from build123d import *
from OCP.BRepFilletAPI import BRepFilletAPI_MakeChamfer

# Parameters (mm, degrees)
SKETCH1_W           = 6.858
SKETCH1_H           = 5.334
BOSS_EXTRUDE1_DEPTH = 4.826
SKETCH2_W           = 1.524
SKETCH2_H           = 1.524
BOSS_EXTRUDE2_DEPTH = 4.826
CHAMFER1_SIZE       = 0.9398
CHAMFER1_SIZE2      = 0.542593783
BOSS_EXTRUDE3_START = -3.048
SKETCH3_W           = 0.720393783
SKETCH3_H           = 1.524
SKETCH3_W_2         = 0.981406217
SKETCH3_W_3         = 1.524
SKETCH3_H_2         = 1.1176
SKETCH3_H_3         = 0.5842
SKETCH3_H_4         = 0.981406217
SKETCH3_H_5         = 0.720393783
BOSS_EXTRUDE3_DEPTH = 0.2032
FILLET2_R           = 0.0508
FILLET3_R           = 0.635
FILLET6_R           = 1.27
SKETCH4_W           = 3.2766
SKETCH4_H           = 3.2258
CUT_EXTRUDE1_DEPTH  = 2.032


with BuildPart() as part:
    # Sketch1 → Boss-Extrude1 (new body)
    with BuildSketch(Plane(origin=(0, 0, 0), x_dir=(1, 0, 0), z_dir=(0, 1, 0))):
        Rectangle(SKETCH1_W, SKETCH1_H)
    extrude(amount=BOSS_EXTRUDE1_DEPTH)

    # Sketch2 → Boss-Extrude2 (add)
    with BuildSketch(Plane(origin=(0, 4.826, 0), x_dir=(1, 0, 0), z_dir=(0, 1, 0))):
        Rectangle(SKETCH2_W, SKETCH2_H)
        with Locations((1.524, 0)):
            Rectangle(SKETCH2_W, SKETCH2_H)
        with Locations((0, 1.524)):
            Rectangle(SKETCH2_W, SKETCH2_H)
        with Locations((-1.524, 0)):
            Rectangle(SKETCH2_W, SKETCH2_H)
        with Locations((0, -1.524)):
            Rectangle(SKETCH2_W, SKETCH2_H)
    extrude(amount=BOSS_EXTRUDE2_DEPTH)

    # Chamfer1: one chamfer whose edges measure the first distance from different faces: ONE call of the kernel's chamfer builder (chamfer() names one face for all edges)
    chamfer1_edges_1 = [part.edges().sort_by_distance(p)[0] for p in [
        (2.286, 9.652, 0),
    ]]
    chamfer1_side_1 = [part.faces().sort_by_distance(p)[0] for p in [
        (2.286, 7.239, 0),
    ]]
    chamfer1_edges_2 = [part.edges().sort_by_distance(p)[0] for p in [
        (0, 9.652, -2.286),
    ]]
    chamfer1_side_2 = [part.faces().sort_by_distance(p)[0] for p in [
        (0, 9.652, 0),
    ]]
    chamfer1_edges_3 = [part.edges().sort_by_distance(p)[0] for p in [
        (-2.286, 9.652, 0),
    ]]
    chamfer1_side_3 = [part.faces().sort_by_distance(p)[0] for p in [
        (-2.286, 7.239, 0),
    ]]
    chamfer1_edges_4 = [part.edges().sort_by_distance(p)[0] for p in [
        (0, 9.652, 2.286),
    ]]
    chamfer1_side_4 = [part.faces().sort_by_distance(p)[0] for p in [
        (0, 7.239, 2.286),
    ]]
    chamfer1 = BRepFilletAPI_MakeChamfer(part.part.solid().wrapped)
    for e in chamfer1_edges_1:
        chamfer1.Add(CHAMFER1_SIZE, CHAMFER1_SIZE2, e.wrapped, chamfer1_side_1[0].wrapped)  # the first distance lies on this face
    for e in chamfer1_edges_2:
        chamfer1.Add(CHAMFER1_SIZE, CHAMFER1_SIZE2, e.wrapped, chamfer1_side_2[0].wrapped)  # the first distance lies on this face
    for e in chamfer1_edges_3:
        chamfer1.Add(CHAMFER1_SIZE, CHAMFER1_SIZE2, e.wrapped, chamfer1_side_3[0].wrapped)  # the first distance lies on this face
    for e in chamfer1_edges_4:
        chamfer1.Add(CHAMFER1_SIZE, CHAMFER1_SIZE2, e.wrapped, chamfer1_side_4[0].wrapped)  # the first distance lies on this face
    add(Compound.cast(chamfer1.Shape()), mode=Mode.REPLACE)

    # Sketch3 → Boss-Extrude3 (add)
    with BuildSketch(Plane(origin=(0, 9.652, 0), x_dir=(1, 0, 0), z_dir=(0, 1, 0)).offset(BOSS_EXTRUDE3_START)):
        with Locations((2.103603109, 0)):
            Rectangle(SKETCH3_W, SKETCH3_H)
        with Locations((1.252703108, 0)):
            Rectangle(SKETCH3_W_2, SKETCH3_H)
        with Locations((0, 1.905)):
            Rectangle(SKETCH3_W_3, SKETCH3_H_2)
        with Locations((0, 1.0541)):
            Rectangle(SKETCH3_W_3, SKETCH3_H_3)
        Rectangle(SKETCH3_W_3, SKETCH3_H)
        with Locations((-1.252703108, 0)):
            Rectangle(SKETCH3_W_2, SKETCH3_H)
        with Locations((-2.103603109, 0)):
            Rectangle(SKETCH3_W, SKETCH3_H)
        with Locations((0, -1.252703108)):
            Rectangle(SKETCH3_W_3, SKETCH3_H_4)
        with Locations((0, -2.103603109)):
            Rectangle(SKETCH3_W_3, SKETCH3_H_5)
    extrude(amount=BOSS_EXTRUDE3_DEPTH)

    # Fillet2
    fillet2_edges = [part.edges().sort_by_distance(p)[0] for p in [
        (-2.4638, 6.8072, 0),
        (0, 6.8072, 2.4638),
        (2.4638, 6.604, 0),
        (2.4638, 6.8072, 0),
        (2.4638, 6.7056, 0.762),
        (2.4638, 6.7056, -0.762),
        (0, 6.8072, -2.4638),
        (0.762, 6.7056, -2.4638),
        (-0.762, 6.7056, -2.4638),
        (-2.4638, 6.604, 0),
        (-2.4638, 6.7056, -0.762),
        (0, 6.604, 2.4638),
        (-0.762, 6.7056, 2.4638),
        (0, 6.604, -2.4638),
        (-2.4638, 6.7056, 0.762),
        (0.762, 6.7056, 2.4638),
    ]]
    fillet(fillet2_edges, radius=FILLET2_R)

    # Fillet3
    fillet3_edges = [part.edges().sort_by_distance(p)[0] for p in [
        (3.429, 2.413, 2.667),
        (-3.429, 2.413, -2.667),
        (3.429, 2.413, -2.667),
    ]]
    fillet(fillet3_edges, radius=FILLET3_R)

    # Fillet6
    fillet6_edges = [part.edges().sort_by_distance(p)[0] for p in [
        (-3.429, 2.413, 2.667),
    ]]
    fillet(fillet6_edges, radius=FILLET6_R)

    # Sketch4 → Cut-Extrude1 (cut)
    with BuildSketch(Plane.XZ):
        Rectangle(SKETCH4_W, SKETCH4_H)
    extrude(amount=-CUT_EXTRUDE1_DEPTH, mode=Mode.SUBTRACT)


solid = part.part
Verification items for the finished model (mm, model axes). A direction names the side the tool comes from. Coordinates: 2 decimals unless noted, no trailing zeros. Loops run counter-clockwise (first coordinate to the right, second up) from the corner with the lowest first, then second, coordinate; pieces in that order, holes last. Notation, with made-up numbers: M 50,77.5 L 55,77.5 A27 cw 55,98.5 Z; hole C -7,49 d3. An arc over 180 degrees is marked long. One line per item, written item: value.
1. Mould release check, pull along Y, two halves, no side actions. Record for faces 1 (the flat face through (2.286, 6, 0)), 2 (the flat face through (-3.429, 2, 0)), 3 (the flat face through (0, 0, -2)): pulls with the +Y half, pulls with the -Y half, needs draft (parallel to the pull), parting line crosses it, or undercut.
Answers follow:
face 1: undercut
face 2: needs draft
face 3: pulls with the -Y half
2. Section check B-B on x = -0.25. Record the cut outline in (y, z).
Answers follow:
outline: M 0,-2.67 L 4.83,-2.67 L 4.83,-2.29 L 6.6,-2.29 L 6.6,-2.41 A0.05 ccw 6.65,-2.46 L 6.76,-2.46 A0.05 ccw 6.81,-2.41 L 6.81,-2.29 L 9.11,-2.29 L 9.65,-1.35 L 9.65,1.74 L 8.71,2.29 L 6.81,2.29 L 6.81,2.41 A0.05 ccw 6.76,2.46 L 6.65,2.46 A0.05 ccw 6.6,2.41 L 6.6,2.29 L 4.83,2.29 L 4.83,2.67 L 0,2.67 L 0,1.61 L 2.03,1.61 L 2.03,-1.61 L 0,-1.61 Z
3. Gauge pin test, flat ends, axial feed: P1, Ø3, axis at x = 0, z = -0.5, coming from the -Y side; P2, Ø0.5, axis at x = -2, y = 7, coming from the +Z side; P3, Ø1.2, axis at y = 6, z = -2, coming from the +X side; P4, Ø0.5, axis at x = 0, y = 6, coming from the +Z side. Record the tip position at first contact, or that the pin passes through.
Answers follow:
P1: y = 0
P2: z = 0.76
P3: x = 0.76
P4: z = 2.29
4. Section check D-D on y = 6.5. Record the cut outline in (x, z).
Answers follow:
outline: M -2.29,-0.76 L -0.76,-0.76 L -0.76,-2.29 L 0.76,-2.29 L 0.76,-0.76 L 2.29,-0.76 L 2.29,0.76 L 0.76,0.76 L 0.76,2.29 L -0.76,2.29 L -0.76,0.76 L -2.29,0.76 Z
5. Material ranges on line 1 along X through (y, z) = (1.75, -0.7); line 2 along Y through (x, z) = (-1.5, -1.75); line 3 along Z through (x, y) = (1, 5.5), recorded low to high. Write a range as from..to.
Answers follow:
line 1: -3.43..-1.64, 1.64..3.43
line 2: 0..4.83
line 3: -0.76..0.76
6. Set-up check for faces 4 (the flat face through (-1.638, 1, 0)), 5 (the flat face through (-2.286, 6, 0)), 6 (the flat face through (0, 8, -2.286)), 7 (the flat face through (0.762, 7, 1)): record each of +Z, -Z, +X, -X, +Y, -Y from which the full face is reachable in a straight line by a thin tool's end or side.
Answers follow:
face 4: -Y
face 5: +Z, -Z, -X
face 6: -Z, +X, -X, +Y
face 7: +Z, +X, +Y
7. Section check C-C on z = -1.8. Record the cut outline in (x, y), plus the area to 3 significant figures.
Answers follow:
outline: M -3.43,0 L 3.43,0 L 3.43,4.83 L 0.76,4.83 L 0.76,9.39 L -0.76,9.39 L -0.76,4.83 L -3.43,4.83 Z
area: 40.1 mm^2
8. Section check A-A on y = 2.5. Record the cut outline in (x, z) (3 decimals), plus the area to 3 significant figures.
Answers follow:
outline: M -3.429,-2.032 A0.635 ccw -2.794,-2.667 L 2.794,-2.667 A0.635 ccw 3.429,-2.032 L 3.429,2.032 A0.635 ccw 2.794,2.667 L -2.159,2.667 A1.27 ccw -3.429,1.397 Z
area: 36.0 mm^2
